Study the drawing (mm; zero at the part's minimum x, y, z) and answer. A direction names the side the tool comes from. Coordinates: 2 decimals unless noted, no trailing zeros. Loops run counter-clockwise (first coordinate to the right, second up) from the corner with the lowest first, then second, coordinate; pieces in that order, holes last. Notation, with made-up numbers: M 34.25,3 L 52.25,3 A25 ccw 52.25,32 Z; hole C -4.5,-30.75 d9. An arc over 180 degrees is marked long. Use one line per item in the form item = value. Start each with the question number.
1. The part is cut by section A-A (x = 7.5). Give the vertices of the cut face in (y, z) (3 decimals).
2. For a pull along Z with two mould halves and no side action, classify the marked faces 1, 2 and 3 as released by +Z, released by -Z, zero draft, split by the parting line, or undercut.
3. A tool of negligible diameter and unlimited length cuts with its end or side. For the marked faces 4 and 5, from which of +Z, -Z, +X, -X, +Y, -Y can it reach the whole face along a straight path? Write none if from no direction.
4. Find the intervals of material crossed by probe 1 along Y at (x, z) = (7.5, 3.5) (3 decimals); probe 2 along Z at (x, y) = (3.5, 1.75); probe 3 along Y at (x, z) = (7.5, 11.25) (3 decimals), in increasing order. Write a range as [from, to].
5. The part is cut by section C-C (z = 14.5). Give the vertices of the cut face in (x, y) (3 decimals), plus the area to 3 significant figures.
6. The part is cut by section B-B (y = 3.25). Give the vertices of the cut face in (x, z), plus the area to 3 significant figures.
7. The part is cut by section D-D (x = 13.5). Give the vertices of the cut face in (y, z).
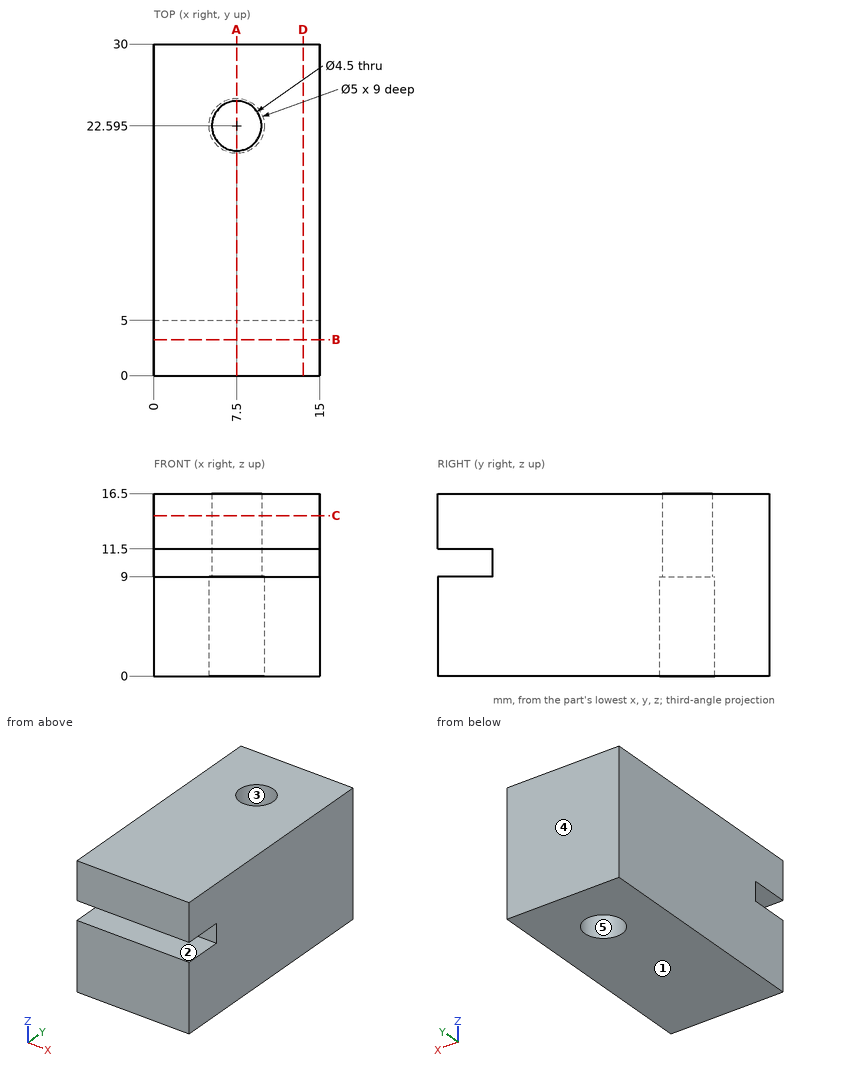
Computed values:
q1.outline = M 0,0 L 20.095,0 L 20.095,9 L 20.345,9 L 20.345,16.5 L 0,16.5 L 0,11.5 L 5,11.5 L 5,9 L 0,9 Z; M 24.845,9 L 25.095,9 L 25.095,0 L 30,0 L 30,16.5 L 24.845,16.5 Z
q2.face_1 = released by -Z
q2.face_2 = undercut
q2.face_3 = zero draft
q3.face_4 = +Z, -Z, +X, -X, +Y
q3.face_5 = -Z
q4.probe_1 = [0, 20.095], [25.095, 30]
q4.probe_2 = [0, 9], [11.5, 16.5]
q4.probe_3 = [5, 20.345], [24.845, 30]
q5.outline = M 0,0 L 15,0 L 15,30 L 0,30 Z; hole C 7.5,22.595 d4.5
q5.area = 434 mm²
q6.outline = M 0,0 L 15,0 L 15,9 L 0,9 Z; M 0,11.5 L 15,11.5 L 15,16.5 L 0,16.5 Z
q6.area = 210 mm²
q7.outline = M 0,0 L 30,0 L 30,16.5 L 0,16.5 L 0,11.5 L 5,11.5 L 5,9 L 0,9 Z
